The model under review builds one solid part; all positions refer to its coordinate system, in mm. A direction names the side the tool comes from. Coordinates: 2 decimals unless noted, no trailing zeros. Loops run counter-clockwise (first coordinate to the right, second up) from the corner with the lowest first, then second, coordinate; pieces in that order, holes last. Notation, with made-up numbers: M 70,52 L 78,52 A13 ccw 78,60 Z; hole C -31,41.5 d7. An arc over 180 degrees is marked long. Use CSV: the item, a comma, the result in double quotes. Start each with the question number.
1. For L1, parallel to X at y = -4.75, z = 1.75; L2, parallel to X at y = -5.5, z = 1.5; L3, parallel to X at y = -5.25, z = 5, list the stretches that pass through material, from the lowest coordinate up.
2. Draft analysis for pull direction X (two halves, no side actions). For faces 5 (the cylindrical face through (-9.66, -2.28, 2.22)), 6 (the flat face through (8, -5, 0)), 7 (the flat face through (-7.62, -5, -3)), state which applies: +X half, -X half, draft (parallel to the pull), parting line (faces both ways), or undercut.
3. Tool access review of faces 1 (the flat face through (11, -3, 4.5)), 2 (the flat face through (-8, -5, 0)), 3 (the flat face through (7.62, -5, -3)), 4 (the flat face through (0, 0, 3)): name each direction out of +Z, -Z, +X, -X, +Y, -Y from which nothing blocks a thin tool from reaching the whole face with its end or side.
4. Add section D-D, the plane z = 4. Write out the cut boundary in (x, y) (1 decimal), then the cut area to 3 significant figures.
5. Clearance check with flat-ended pins moving along their axes: P1, Ø3.5, axis at x = 11.5, y = -6.5, coming from the -Z side; P2, Ø8, axis at x = -1.5, z = -4, coming from the +Y side; P3, Ø5.5, axis at y = -4.5, z = -3, coming from the -X side; P4, Ø1.7, axis at x = 10, y = -4, coming from the -Z side. State where each tip first meets the part, or that it passes through.
6. Add section A-A, the plane z = 2. Write out the cut boundary in (x, y) (1 decimal).
7. Add section B-B, the plane y = -0.75. Write out the cut boundary in (x, z), then the cut area to 3 significant figures.
8. Add section C-C, the plane x = -10. Write out the cut boundary in (y, z) (3 decimals), then the cut area to 3 significant figures.
from build123d import *

# Parameters (mm, degrees)
F1_DEPTH = 9.525
F2_R     = 1.6
F3_DEPTH = 10
F4_R     = 2.54
F5_R     = 2.8
F6_DEPTH = 4.5


with BuildPart() as f1:
    # F0 (on Front) → F1 (new body)
    with BuildSketch(Plane.XZ):
        with BuildLine():
            Line((-14.2875, 10), (-14.2875, 0))
            Line((-14.2875, 0), (-7.62, 0))
            Line((-7.62, 0), (-7.62, -7.62))
            Line((-7.62, -7.62), (0, -7.62))
            Line((0, -7.62), (0, -4.9395))
            ThreePointArc((0, -4.9395), (-3.6695, -1.27), (0, 2.3995))
            Line((0, 2.3995), (0, 10))
            Line((0, 10), (-14.2875, 10))
        make_face()
        with BuildLine():
            Line((14.2875, 10), (0, 10))
            Line((0, 10), (0, 2.3995))
            ThreePointArc((0, 2.3995), (2.594728, 1.324728), (3.6695, -1.27))
            ThreePointArc((3.6695, -1.27), (2.594728, -3.864728), (0, -4.9395))
            Line((0, -4.9395), (0, -7.62))
            Line((0, -7.62), (7.62, -7.62))
            Line((7.62, -7.62), (7.62, 0))
            Line((7.62, 0), (14.2875, 0))
            Line((14.2875, 0), (14.2875, 10))
        make_face()
    extrude(amount=F1_DEPTH)

    # F2 (on face) → F3 (cut, through all)
    with BuildSketch(Plane(origin=(0, 0, 0), x_dir=(1, 0, 0), z_dir=(0, 0, -1))):
        with BuildLine():
            Line((-10.95375, 4.7625), (-9.35375, 4.7625))
            ThreePointArc((-9.35375, 4.7625), (-9.822379, 5.893871), (-10.95375, 6.3625))
            Line((-10.95375, 6.3625), (-10.95375, 4.7625))
        make_face()
        with BuildLine():
            ThreePointArc((-10.95375, 3.1625), (-9.822379, 3.631129), (-9.35375, 4.7625))
            Line((-9.35375, 4.7625), (-10.95375, 4.7625))
            Line((-10.95375, 4.7625), (-10.95375, 3.1625))
        make_face()
        with BuildLine():
            Line((-10.95375, 4.7625), (-10.95375, 6.3625))
            ThreePointArc((-10.95375, 6.3625), (-12.085121, 5.893871), (-12.55375, 4.7625))
            Line((-12.55375, 4.7625), (-10.95375, 4.7625))
        make_face()
        with BuildLine():
            ThreePointArc((-12.55375, 4.7625), (-12.085121, 3.631129), (-10.95375, 3.1625))
            Line((-10.95375, 3.1625), (-10.95375, 4.7625))
            Line((-10.95375, 4.7625), (-12.55375, 4.7625))
        make_face()
        with Locations((10.95375, 4.7625)):
            Circle(F2_R)
    extrude(amount=-F3_DEPTH, mode=Mode.SUBTRACT)

    # F4
    f4_edges = [f1.edges().sort_by_distance(p)[0] for p in [
        (-7.62, -4.7625, -7.62),
        (7.62, -4.7625, -7.62),
    ]]
    fillet(f4_edges, radius=F4_R)

    # F5 (on face) → F6 (cut)
    with BuildSketch(Plane(origin=(0, 0, 0), x_dir=(1, 0, 0), z_dir=(0, 0, -1))):
        with Locations((-10.95375, 4.7625)):
            Circle(F5_R)
        with Locations((10.95375, 4.7625)):
            Circle(F5_R)
    extrude(amount=-F6_DEPTH, mode=Mode.SUBTRACT)


solid = f1.part
Computed:
1,L1,"x = -14.29 to -13.75, -8.15 to -2.08, 2.08 to 8.15, 13.75 to 14.29"
1,L2,"x = -14.29 to -13.65, -8.25 to -2.41, 2.41 to 8.25, 13.65 to 14.29"
1,L3,"x = -14.29 to -12.48, -9.43 to 9.43, 12.48 to 14.29"
2,face 5,"undercut"
2,face 6,"draft"
2,face 7,"-X half"
3,face 1,"-Z"
3,face 2,"-Z, -X, +Y, -Y"
3,face 3,"-Z, +X, +Y, -Y"
3,face 4,"+Z, -Z, +X, -X, +Y"
4,outline,"M -14.3,-9.5 L 14.3,-9.5 L 14.3,0 L -14.3,0 Z; hole C -11,-4.8 d5.6; hole C 11,-4.8 d5.6"
4,area,"223 mm^2"
5,P1,"stops at z = 0"
5,P2,"stops at y = 0"
5,P3,"stops at x = -7.62"
5,P4,"stops at z = 4.5"
6,outline,"M -14.3,-9.5 L -1.7,-9.5 L -1.7,0 L -14.3,0 Z; M 1.7,-9.5 L 14.3,-9.5 L 14.3,0 L 1.7,0 Z; hole C -11,-4.8 d5.6; hole C 11,-4.8 d5.6"
7,outline,"M -14.29,0 L -7.62,0 L -7.62,-5.08 A2.54 ccw -5.08,-7.62 L 5.08,-7.62 A2.54 ccw 7.62,-5.08 L 7.62,0 L 14.29,0 L 14.29,10 L -14.29,10 Z; hole M 0,-4.94 A3.67 ccw 3.67,-1.27 A3.67 ccw 0,2.4 A3.67 ccw Z"
7,area,"357 mm^2"
8,outline,"M -9.525,0 L -7.395,0 L -7.395,4.5 L -6.047,4.5 L -6.047,10 L -9.525,10 Z; M -3.478,4.5 L -2.13,4.5 L -2.13,0 L 0,0 L 0,10 L -3.478,10 Z"
8,area,"57.4 mm^2"
